CAD build for the part. Positions are in the model's coordinates, mm. A direction names the side the tool comes from. Coordinates: 2 decimals unless noted, no trailing zeros. Order: outer loops, then holes, each group sorted by start corner. A loop starts at its lowest first (then second) coordinate and runs counter-clockwise, first axis right, second up. Notation, with made-up numbers: (36.5, -36.5) - (77.5, -36.5) arc R24 ccw to (77.5, 1.5) - close; hole circle Ø2 at (47.25, -20.75). An arc over 180 degrees is marked (long way). Return JSON: item names as keys, results as strings.
from build123d import *

# Parameters (mm, degrees)
F0_W      = 1079.5
F0_H      = 762
F1_DEPTH  = 1600.2
F3_DEPTH  = 2032
F4_W      = 228.6
F4_H      = 25.4
F5_DEPTH  = 889
F6_W      = 228.6
F6_H      = 25.4
F7_DEPTH  = 762
F9_DEPTH  = 2032
F10_R     = 44.45
F11_DEPTH = 76.2
F12_R     = 76.2
F12_R_2   = 44.45
F13_DEPTH = 12.7
F14_R     = 9.0043
F14_R_2   = 20.8788
F15_DEPTH = 25.4


with BuildPart() as f1:
    # F0 (on Front) → F1 (new body)
    with BuildSketch(Plane.XZ):
        Rectangle(F0_W, F0_H)
    extrude(amount=F1_DEPTH)

    # F2 (on face) → F3 (cut)
    with BuildSketch(Plane.XZ.offset(1600.2)):
        with BuildLine():
            Line((-539.75, 381), (-539.75, 266.7))
            Line((-539.75, 266.7), (-311.15, 266.7))
            ThreePointArc((-311.15, 266.7), (-181.819542348, 349.0410030714), (-31.8694487214, 381))
            Line((-31.8694487214, 381), (-539.75, 381))
        make_face()
        with BuildLine():
            Line((539.75, 381), (63.2200438553, 381))
            ThreePointArc((63.2200438553, 381), (196.4561263356, 343.9601006936), (311.15, 266.7))
            Line((311.15, 266.7), (539.75, 266.7))
            Line((539.75, 266.7), (539.75, 381))
        make_face()
        with BuildLine():
            ThreePointArc((311.15, -266.7), (183.8275613975, -348.3038933111), (36.1753911372, -381))
            Line((36.1753911372, -381), (539.75, -381))
            Line((539.75, -381), (539.75, -266.7))
            Line((539.75, -266.7), (311.15, -266.7))
        make_face()
        with BuildLine():
            Line((-311.15, -266.7), (-539.75, -266.7))
            Line((-539.75, -266.7), (-539.75, -381))
            Line((-539.75, -381), (-36.1753911372, -381))
            ThreePointArc((-36.1753911372, -381), (-183.8275613975, -348.3038933111), (-311.15, -266.7))
        make_face()
    extrude(amount=-F3_DEPTH, mode=Mode.SUBTRACT)

    # F4 (on face) → F5 (cut)
    with BuildSketch(Plane.XY.offset(266.7)):
        with Locations((-425.45, -1358.9)):
            Rectangle(F4_W, F4_H)
        with Locations((-425.45, -1104.9)):
            Rectangle(F4_W, F4_H)
        with Locations((-425.45, -850.9)):
            Rectangle(F4_W, F4_H)
        with Locations((-425.45, -596.9)):
            Rectangle(F4_W, F4_H)
        with Locations((-425.45, -342.9)):
            Rectangle(F4_W, F4_H)
    extrude(amount=-F5_DEPTH, mode=Mode.SUBTRACT)

    # F6 (on face) → F7 (cut)
    with BuildSketch(Plane.XY.offset(266.7)):
        with Locations((425.45, -1358.9)):
            Rectangle(F6_W, F6_H)
        with Locations((425.45, -1104.9)):
            Rectangle(F6_W, F6_H)
        with Locations((425.45, -850.9)):
            Rectangle(F6_W, F6_H)
        with Locations((425.45, -596.9)):
            Rectangle(F6_W, F6_H)
        with Locations((425.45, -342.9)):
            Rectangle(F6_W, F6_H)
    extrude(amount=-F7_DEPTH, mode=Mode.SUBTRACT)

    # F8 (on face) → F9 (cut)
    with BuildSketch(Plane.XZ.offset(1600.2)):
        with BuildLine():
            ThreePointArc((-539.75, 228.6), (-528.5907683632, 255.5407683632), (-501.65, 266.7))
            Line((-501.65, 266.7), (-539.75, 266.7))
            Line((-539.75, 266.7), (-539.75, 228.6))
        make_face()
        with BuildLine():
            ThreePointArc((-501.65, -266.7), (-528.5907683632, -255.5407683632), (-539.75, -228.6))
            Line((-539.75, -228.6), (-539.75, -266.7))
            Line((-539.75, -266.7), (-501.65, -266.7))
        make_face()
        with BuildLine():
            Line((539.75, -266.7), (539.75, -228.6))
            ThreePointArc((539.75, -228.6), (528.5907683632, -255.5407683632), (501.65, -266.7))
            Line((501.65, -266.7), (539.75, -266.7))
        make_face()
        with BuildLine():
            Line((539.75, 266.7), (501.65, 266.7))
            ThreePointArc((501.65, 266.7), (528.5907683632, 255.5407683632), (539.75, 228.6))
            Line((539.75, 228.6), (539.75, 266.7))
        make_face()
    extrude(amount=-F9_DEPTH, mode=Mode.SUBTRACT)

    # F10 (on face) → F11 (join)
    with BuildSketch(Plane.XZ.offset(1600.2)):
        Circle(F10_R)
    extrude(amount=F11_DEPTH)

    # F12 (on face) → F13 (join)
    with BuildSketch(Plane.XZ.offset(1676.4)):
        Circle(F12_R)
        Circle(F12_R_2, mode=Mode.SUBTRACT)
        Circle(F12_R_2)
    extrude(amount=F13_DEPTH)

    # F14 (on face) → F15 (cut)
    with BuildSketch(Plane.XZ.offset(1689.1)):
        with Locations((-28.9941, 50.2192543197)):
            Circle(F14_R)
        with Locations((-57.9882, 0)):
            Circle(F14_R)
        with Locations((-28.9941, -50.2192543197)):
            Circle(F14_R)
        with Locations((29.0321442983, -50.2412)):
            Circle(F14_R)
        with Locations((57.9882, 0)):
            Circle(F14_R)
        with Locations((28.9941, 50.2192543197)):
            Circle(F14_R)
        Circle(F14_R_2)
    extrude(amount=-F15_DEPTH, mode=Mode.SUBTRACT)


solid = f1.part
Item 1: Drop flat-ended pins along their axis: P1, Ø1, axis at x = -138.5, z = -231, coming from the +Y side; P2, Ø7.5, axis at y = -1101.5, z = 100, coming from the -X side; P3, Ø10, axis at x = -3, z = -120, coming from the -Y side; P4, Ø6, axis at x = -378.5, y = -367.5, coming from the -Z side. Give the stop position or say it passes through.
Findings below:
{"P1": "stops at y = 0", "P2": "stops at x = -311.15", "P3": "stops at y = -1600.2", "P4": "stops at z = -266.7"}
Item 2: Mould opens along Y. For faces 4 (the flat face through (424, -1092.2, 4)), 5 (the flat face through (424, -330.2, 4)), 6 (the cylindrical face through (-528.89, -979.5, 255.24)) say: released by +Y, released by -Y, zero draft, split by the parting line, or undercut.
Findings below:
{"face 4": "undercut", "face 5": "undercut", "face 6": "zero draft"}
Item 3: Band-saw the part on B-B, the plane y = -996.5. List the corners of the cut face in (x, z), then the cut area to 3 significant figures.
Findings below:
{"outline": "(-539.75, -228.6) arc R38.1 ccw to (-501.65, -266.7) - (-311.15, -266.7) arc R431.8 ccw to (-36.18, -381) - (36.18, -381) arc R431.8 ccw to (311.15, -266.7) - (501.65, -266.7) arc R38.1 ccw to (539.75, -228.6) - (539.75, 228.6) arc R38.1 ccw to (501.65, 266.7) - (311.15, 266.7) arc R431.8 ccw to (63.22, 381) - (-31.87, 381) arc R431.8 ccw to (-311.15, 266.7) - (-501.65, 266.7) arc R38.1 ccw to (-539.75, 228.6) - close", "area": "675,000 mm²"}
Item 4: Wall check: L1, parallel to Y at x = -360.5, z = 203; L2, parallel to Z at x = 0, y = -1683; L3, parallel to Y at x = 215, z = -169.5. Give the ranges that are in metal, low to high. Write a range as [from, to].
Findings below:
{"L1": "y = [-1600.2, -1371.6], [-1346.2, -1117.6], [-1092.2, -863.6], [-838.2, -609.6], [-584.2, -355.6], [-330.2, 0]", "L2": "z = [-76.2, -20.88], [20.88, 76.2]", "L3": "y = [-1600.2, 0]"}
Item 5: Band-saw the part on A-A, the plane x = 0. List the corners of the cut face in (y, z), then the cut area to 3 significant figures.
Findings below:
{"outline": "(-1689.1, -76.2) - (-1676.4, -76.2) - (-1676.4, -44.45) - (-1600.2, -44.45) - (-1600.2, -381) - (0, -381) - (0, 381) - (-1600.2, 381) - (-1600.2, 44.45) - (-1676.4, 44.45) - (-1676.4, 76.2) - (-1689.1, 76.2) - (-1689.1, 20.88) - (-1663.7, 20.88) - (-1663.7, -20.88) - (-1689.1, -20.88) - close", "area": "1,230,000 mm²"}
Item 6: Which spindle directions (+Z, -Z, +X, -X, +Y, -Y) get a long thin tool onto all of the face, cutting with end or side? Do faces 1 (the flat face through (424, -1117.6, 4)), 2 (the flat face through (-408, -167, 266.7)), 3 (the flat face through (-427, -1117.6, 4)). Say none if no direction does.
Findings below:
{"face 1": "+Z, -Z, +X", "face 2": "+Z, -X, +Y, -Y", "face 3": "+Z, -Z, -X"}
